Part model, mm, in its own coordinate system. Coordinates: 2 decimals unless noted, no trailing zeros. Loops run counter-clockwise (first coordinate to the right, second up) from the corner with the lowest first, then second, coordinate; pieces in that order, holes last. Notation, with made-up numbers: (-29, 62.5) - (-19, 62.5) arc R23 cw to (-19, 97.5) - close; hole circle Ø3 at (35.25, -24.5). An arc over 180 degrees is marked (long way). Use a Markdown table: item, result. Add a question column.
1) Pull direction Z, two halves, no side cores. Call faces 1 (the face through (-27.39, -0.36, 361.34)), 2 (the face through (-7, 0, 0)), 3 (the face through (-50.8, 0, 169)), 4 (the face through (4, 0, 375.907)): +Z half, -Z half, draft (parallel to the pull), parting line (faces both ways), or undercut.
2) Probe probe 1 along Z at (x, y) = (-39, 17.5); probe 2 along Z at (x, y) = (-29.5, -22). List the from-to ranges inside material, lowest first. Write a range as [from, to].
3) Band-saw the part on B-B (x = -40). Give the cut face in (y, z), plus the area to 3 significant figures.
4) Drop a flat-ended pin along its axis: P1, Ø8, axis at x = -34.5, y = 18, coming from the +Z side. Give the stop position or say it passes through.
5) Band-saw the part on A-A (y = 17.5). Give the cut face in (x, z).
from build123d import *

# Parameters (mm, degrees)
SKETCH1_W               = 101.6
SKETCH1_H               = 50.8
BOSS_EXTRUDE1_DEPTH     = 375.907215418
CUT_EXTRUDE1_DEPTH      = 383.710745346
CUT_EXTRUDE1_DEPTH_BACK = 383.710745346
CUT_EXTRUDE2_DEPTH      = 383.710745346
CUT_EXTRUDE2_DEPTH_BACK = 383.710745346
SKETCH3_W               = 12.7
SKETCH3_H               = 375.907215418


with BuildPart() as part:
    # Sketch1 → Boss-Extrude1 (new body)
    with BuildSketch(Plane.XY):
        Rectangle(SKETCH1_W, SKETCH1_H)
    extrude(amount=BOSS_EXTRUDE1_DEPTH)

    # Sketch2 → Cut-Extrude1 (cut, two sides: drawn at the far end of the back side and taken through both)
    with BuildSketch(Plane(origin=(0, 25.4, 0), x_dir=(1, 0, 0), z_dir=(0, 1, 0)).offset(-CUT_EXTRUDE1_DEPTH_BACK)):
        Polygon((-50.8, -343.610078217), (-25.4, -347.179815418), (-29.437372775, -375.907215418), (-50.8, -375.907215418), align=None)
    extrude(amount=CUT_EXTRUDE1_DEPTH + CUT_EXTRUDE1_DEPTH_BACK, mode=Mode.SUBTRACT)

    # Sketch3 → Cut-Extrude2 (cut, two sides: drawn at the far end of the back side and taken through both)
    with BuildSketch(Plane(origin=(0, 25.4, 0), x_dir=(1, 0, 0), z_dir=(0, 1, 0)).offset(-CUT_EXTRUDE2_DEPTH_BACK)):
        with Locations((44.45, -187.953607709)):
            Rectangle(SKETCH3_W, SKETCH3_H)
    extrude(amount=CUT_EXTRUDE2_DEPTH + CUT_EXTRUDE2_DEPTH_BACK, mode=Mode.SUBTRACT)


solid = part.part
Answer block:
| question | item | result |
|---|---|---|
| 1 | face 1 | undercut |
| 1 | face 2 | -Z half |
| 1 | face 3 | draft |
| 1 | face 4 | +Z half |
| 2 | probe 1 | [0, 345.27] |
| 2 | probe 2 | [0, 346.6] |
| 3 | outline | (-25.4, 0) - (25.4, 0) - (25.4, 345.13) - (-25.4, 345.13) - close |
| 3 | area | 17,500 mm2 |
| 4 | P1 | z = 346.46 |
| 5 | outline | (-50.8, 0) - (38.1, 0) - (38.1, 375.91) - (-29.44, 375.91) - (-25.4, 347.18) - (-50.8, 343.61) - close |
